from build123d import *

# Parameters (mm, degrees)
F1_DEPTH = 30
F2_DEPTH = 20
F3_DEPTH = 20
F4_DEPTH = 15


with BuildPart() as f1:
    # F0 (on Top) → F1 (new body)
    with BuildSketch(Plane.XY):
        with BuildLine():
            ThreePointArc((0, 9), (6.3639610307, 6.3639610307), (9, 0))
            ThreePointArc((9, 0), (6.3639610307, -6.3639610307), (0, -9))
            Line((0, -9), (0, -9.5))
            ThreePointArc((0, -9.5), (6.7175144213, -6.7175144213), (9.5, 0))
            ThreePointArc((9.5, 0), (6.7175144213, 6.7175144213), (0, 9.5))
            Line((0, 9.5), (0, 9))
        make_face()
        with BuildLine():
            ThreePointArc((0, -9), (-9, 0), (0, 9))
            Line((0, 9), (0, 9.5))
            ThreePointArc((0, 9.5), (-9.5, 0), (0, -9.5))
            Line((0, -9.5), (0, -9))
        make_face()
        with BuildLine():
            Line((100, 9.5), (0, 9.5))
            ThreePointArc((0, 9.5), (6.7175144213, 6.7175144213), (9.5, 0))
            ThreePointArc((9.5, 0), (6.7175144213, -6.7175144213), (0, -9.5))
            Line((0, -9.5), (100, -9.5))
            Line((100, -9.5), (100, 9.5))
        make_face()
    extrude(amount=F1_DEPTH)

    # F0 (on Top) → F2 (join)
    with BuildSketch(Plane.XY):
        with BuildLine():
            Line((100, 9.5), (0, 9.5))
            ThreePointArc((0, 9.5), (6.7175144213, 6.7175144213), (9.5, 0))
            ThreePointArc((9.5, 0), (6.7175144213, -6.7175144213), (0, -9.5))
            Line((0, -9.5), (100, -9.5))
            Line((100, -9.5), (100, 9.5))
        make_face()
        with BuildLine():
            ThreePointArc((0, 9), (6.3639610307, 6.3639610307), (9, 0))
            ThreePointArc((9, 0), (6.3639610307, -6.3639610307), (0, -9))
            Line((0, -9), (0, -9.5))
            ThreePointArc((0, -9.5), (6.7175144213, -6.7175144213), (9.5, 0))
            ThreePointArc((9.5, 0), (6.7175144213, 6.7175144213), (0, 9.5))
            Line((0, 9.5), (0, 9))
        make_face()
        with BuildLine():
            ThreePointArc((0, -9), (6.3639610307, -6.3639610307), (9, 0))
            ThreePointArc((9, 0), (6.3639610307, 6.3639610307), (0, 9))
            Line((0, 9), (0, 0))
            Line((0, 0), (0, -9))
        make_face()
        with BuildLine():
            ThreePointArc((0, -9), (-9, 0), (0, 9))
            Line((0, 9), (0, 9.5))
            ThreePointArc((0, 9.5), (-9.5, 0), (0, -9.5))
            Line((0, -9.5), (0, -9))
        make_face()
        with BuildLine():
            Line((0, 0), (0, 9))
            ThreePointArc((0, 9), (-9, 0), (0, -9))
            Line((0, -9), (0, 0))
        make_face()
    extrude(amount=-F2_DEPTH)

    # F3 (add): a face of the model
    f3_faces = [f1.faces().sort_by_distance(p)[0] for p in [
        (50, 9.5, 5),
    ]]
    extrude(f3_faces, amount=F3_DEPTH)

    # F4 (cut): a face of the model
    f4_faces = [f1.faces().sort_by_distance(p)[0] for p in [
        (48.1048371306, 9.6492512785, -20),
    ]]
    extrude(f4_faces, amount=-F4_DEPTH, mode=Mode.SUBTRACT)


solid = f1.part
Model file for the job. Use its own axes, mm. A direction names the side the tool comes from. Give positions to 0.01 mm unless a question says otherwise; leave off trailing zeros. Write each loop counter-clockwise with the first axis right and the second up, starting at its lowest first coordinate (ties: lowest second). Pieces come first, ordered by that corner, then holes. Notation, with made-up numbers: M 11,41.5 L 23,41.5 A16 cw 23,69.5 Z; hole C 59.25,42 d2. An arc over 180 degrees is marked long. One line per item, written item: value. Start each with the question number.
Q1. 3-axis set-ups, long thin cutter, end or side, ignore diameter. For faces 1 (the flat face through (0, 19, 12)), 2 (the flat face through (58, 10, 30)): which of +Z, -Z, +X, -X, +Y, -Y reach the whole face in a straight line?
Q2. Two-plate mould, pull along Y, no slides. Class faces 3 (the flat face through (100, 10, 13)), 4 (the flat face through (0, 0, 0)), 5 (the flat face through (51, 29.5, 13)), 6 (the flat face through (49, -9.5, 13)): +Y half, -Y half, draft (parallel to the pull), parting line (faces both ways), or undercut.
Q3. Saw through at C-C, the plane y = 4. Write the cut outline in (x, z), plus the area to 3 significant figures.
Q4. Drop flat-ended pins along their axis: pin 1 Ø1 at (y, z) = (12, 18.5) entering from -X; pin 2 Ø2 at (y, z) = (7.5, 10.5) entering from -X; pin 3 Ø5.5 at (x, y) = (2, -2) entering from +Z. Give the stop position or say it passes through.
Q5. Probe probe 1 along X at (y, z) = (-7, 13.5); probe 2 along Z at (x, y) = (2, 4); probe 3 along X at (y, z) = (17.5, 19.5). List the from-to ranges inside material, lowest first. Write a range as [from, to].
Q6. Saw through at B-B, the plane z = 25.5. Write the cut outline in (x, y), plus the area to 3 significant figures.
Q7. Saw through at A-A, the plane z = -1.5. Write the cut outline in (x, y), plus the area to 3 significant figures.
Q8. Saw through at D-D, the plane y = 11. Write the cut outline in (x, z).
Output values:
1. face 1: +Z, -Z, -X, +Y
1. face 2: +Z, +X, -X, +Y, -Y
2. face 3: draft
2. face 4: undercut
2. face 5: +Y half
2. face 6: -Y half
3. outline: M -8.62,-5 L 100,-5 L 100,30 L 8.06,30 L 8.06,0 L -8.06,0 L -8.06,30 L -8.62,30 Z
3. area: 3,320 mm²
4. pin 1: stops at x = 0
4. pin 2: stops at x = -6.93
4. pin 3: stops at z = 0
5. probe 1: x = [-6.42, -5.66], [5.66, 100]
5. probe 2: z = [-5, 0]
5. probe 3: x = [0, 100]
6. outline: M 0,-9.5 L 100,-9.5 L 100,29.5 L 0,29.5 L 0,9.5 A9.5 ccw Z; hole C 0,0 d18
6. area: 3,790 mm²
7. outline: M 0,-9.5 L 100,-9.5 L 100,29.5 L 0,29.5 L 0,9.5 A9.5 ccw Z
7. area: 4,040 mm²
8. outline: M 0,-5 L 100,-5 L 100,30 L 0,30 Z
